from build123d import *

# Parameters (mm, degrees)
SKETCH1_W           = 40
SKETCH1_H           = 50
SKETCH1_W_2         = 12.5
SKETCH1_H_2         = 20
BOSS_EXTRUDE1_DEPTH = 2.5
SKETCH2_R           = 1.5
CUT_EXTRUDE1_DEPTH  = 10
SKETCH3_R           = 3.75
CUT_EXTRUDE2_DEPTH  = 1
CHAMFER1_SIZE       = 2.5


with BuildPart() as part:
    # Sketch1 → Boss-Extrude1 (new body)
    with BuildSketch(Plane(origin=(0, 0, 0), x_dir=(1, 0, 0), z_dir=(0, 1, 0))):
        Rectangle(SKETCH1_W, SKETCH1_H)
        with Locations((-8.25, 0)):
            Rectangle(SKETCH1_W_2, SKETCH1_H_2, mode=Mode.SUBTRACT)
        with Locations((8.25, 0)):
            Rectangle(SKETCH1_W_2, SKETCH1_H_2, mode=Mode.SUBTRACT)
    extrude(amount=BOSS_EXTRUDE1_DEPTH)

    # Sketch2 → Cut-Extrude1 (cut)
    with BuildSketch(Plane(origin=(0, 2.5, 0), x_dir=(1, 0, 0), z_dir=(0, 1, 0))):
        with Locations(Location((0, 17.5, 0), (0, 0, 270))):
            Circle(SKETCH2_R)
        with Locations(Location((0, -17.5, 0), (0, 0, 270))):
            Circle(SKETCH2_R)
    extrude(amount=-CUT_EXTRUDE1_DEPTH, mode=Mode.SUBTRACT)

    # Sketch3 → Cut-Extrude2 (cut)
    with BuildSketch(Plane(origin=(0, 2.5, 0), x_dir=(1, 0, 0), z_dir=(0, 1, 0))):
        with Locations(Location((0, 17.5, 0), (0, 0, 270))):
            Circle(SKETCH3_R)
        with Locations(Location((0, -17.5, 0), (0, 0, 270))):
            Circle(SKETCH3_R)
    extrude(amount=-CUT_EXTRUDE2_DEPTH, mode=Mode.SUBTRACT)

    # Chamfer1
    chamfer1_edges = [part.edges().sort_by_distance(p)[0] for p in [
        (20, 2.5, 0),
        (0, 2.5, 25),
        (0, 2.5, -25),
        (-20, 2.5, 0),
    ]]
    chamfer(chamfer1_edges, length=CHAMFER1_SIZE - 0.0001)  # a hair under: the kernel refuses the full size


solid = part.part
Here's how the part is built. I have some questions about the finished solid (model axes, mm). A direction names the side the tool comes from. Round coordinates to 2 decimals unless told otherwise and drop trailing zeros. Write each question's results on one line, items separated by ' | '.
(1) We'd pull the mould along X, two halves only. Please class faces 1 (the face through (0, 1, 24)), 2 (the face through (19, 1, 0)), 3 (the face through (8, 1, 10)): released by +X, released by -X, zero draft, split by the parting line, or undercut.
Worked answers:
face 1: zero draft | face 2: released by +X | face 3: undercut
(2) If we section it at B-B, the plane z = 2: Give the number of separate pieces and of enclosed holes in the cut face, then the cut area to 3 significant figures.
Worked answers:
separate pieces: 3 | enclosed holes: 0 | area: 31.3 mm2
(3) For P1, Ø1.2, axis at y = 1, z = 2, coming from the -X side; P2, Ø1.5, axis at x = -15.5, y = 0.5, coming from the -Z side; P3, Ø8, axis at x = -1, z = 17.5, coming from the +Y side; P4, Ø1.2, axis at x = -8, y = 1.5, coming from the -Z side, each with a flat end and sliding along its axis, tell me the tip position at first contact or that it passes through.
Worked answers:
P1: x = -19.6 | P2: z = -25 | P3: y = 2.5 | P4: z = -24.1
(4) For faces 4 (the face through (0, 0, 0)), 5 (the face through (-8, 1, -10)), 6 (the face through (0.165, 2.007, 13.754)), which set-ups out of +Z, -Z, +X, -X, +Y, -Y let a thin tool reach every point of the face, with its end or its side?
Worked answers:
face 4: +Z, -Z, +X, -X, -Y | face 5: +Y, -Y | face 6: +Y
(5) If I drill on L1, parallel to X at y = 1.8, z = 3.5; L2, parallel to Y at x = -18, z = -18; L3, parallel to Z at x = -11.5, y = 0.75, over which ranges is the centre line in solid material (lowest first)?
Worked answers:
L1: -18.2 to -14.5, -2 to 2, 14.5 to 18.2 | L2: 0 to 2 | L3: -24.25 to -10, 10 to 24.25
